from build123d import *

# Parameters (mm, degrees)
SKETCH1_W           = 120
SKETCH1_H           = 120
BOSS_EXTRUDE1_DEPTH = 10
SKETCH2_R           = 45
BOSS_EXTRUDE2_DEPTH = 40
SKETCH3_W           = 10
SKETCH3_H           = 80
BOSS_EXTRUDE3_DEPTH = 50
SKETCH4_R           = 20
BOSS_EXTRUDE4_DEPTH = 25
FILLET1_R           = 2
SKETCH6_R           = 6
BOSS_EXTRUDE5_DEPTH = 2
SKETCH7_R           = 5
BOSS_EXTRUDE6_DEPTH = 30


with BuildPart() as part:
    # Sketch1 → Boss-Extrude1 (new body)
    with BuildSketch(Plane.XY):
        Rectangle(SKETCH1_W, SKETCH1_H)
    extrude(amount=BOSS_EXTRUDE1_DEPTH)

    # Sketch3 → Boss-Extrude3 (add)
    with BuildSketch(Plane(origin=(0, 0, 0), x_dir=(-1, 0, 0), z_dir=(0, 0, -1))):
        with Locations((-25, 0)):
            Rectangle(SKETCH3_W, SKETCH3_H)
        with Locations((25, 0)):
            Rectangle(SKETCH3_W, SKETCH3_H)
    extrude(amount=BOSS_EXTRUDE3_DEPTH)



with BuildPart() as body_2:
    # Sketch2 → Boss-Extrude2 (new body, symmetric)
    with BuildSketch(Plane(origin=(0, 0, 0), x_dir=(1, 0, 0), z_dir=(0, 1, 0))):
        with Locations((0, 50)):
            Circle(SKETCH2_R)
    extrude(amount=BOSS_EXTRUDE2_DEPTH, both=True)


with BuildPart() as part_1:
    add(part.part)

    add(body_2.part)  # Boss-Extrude4 merges body 2
    # Sketch4 → Boss-Extrude4 (add)
    with BuildSketch(Plane(origin=(0, 40, 0), x_dir=(1, 0, 0), z_dir=(0, 1, 0))):
        with Locations((0, 50)):
            Circle(SKETCH4_R)
    extrude(amount=BOSS_EXTRUDE4_DEPTH)

    # Fillet1
    fillet1_edges = [part_1.edges().sort_by_distance(p)[0] for p in [
        (-20, 40, -50),
    ]]
    fillet(fillet1_edges, radius=FILLET1_R)

    # Sketch6 → Boss-Extrude5 (add)
    with BuildSketch(Plane(origin=(0, 65, 0), x_dir=(1, 0, 0), z_dir=(0, 1, 0))):
        with Locations((0, 50)):
            Circle(SKETCH6_R)
    extrude(amount=BOSS_EXTRUDE5_DEPTH)

    # Sketch7 → Boss-Extrude6 (add)
    with BuildSketch(Plane(origin=(0, 67, 0), x_dir=(1, 0, 0), z_dir=(0, 1, 0))):
        with Locations((0, 50)):
            Circle(SKETCH7_R)
    extrude(amount=BOSS_EXTRUDE6_DEPTH)


solid = part_1.part
The listing builds one solid part. Answer for the finished solid, in the listing's coordinates (mm). A direction names the side the tool comes from. Coordinates: 2 decimals unless noted, no trailing zeros. Loops run counter-clockwise (first coordinate to the right, second up) from the corner with the lowest first, then second, coordinate; pieces in that order, holes last. Notation, with made-up numbers: (51.25, 57) -> (64.25, 57) arc R24 ccw to (64.25, 79) -> close; hole circle Ø6 at (76, 58). An arc over 180 degrees is marked (long way). Answer in a Markdown table with one row per item. Add a question column.
1. The part is cut by section D-D, the plane z = -50. Write down the section's boundary in (x, y).
2. Flat-ended cylindrical pins translate along their axes: P1, Ø5, axis at x = -12.5, z = -83.5, coming from the -Y side; P2, Ø3, axis at y = 15.5, z = -81.5, coming from the +X side; P3, Ø10.5, axis at y = 17.5, z = -6.5, coming from the -X side. Find the tip coordinate at first contact, or state that the pin passes through.
3. The part is cut by section C-C, the plane y = 0. Write down the section's boundary in (x, z).
4. Determine the mould class of faces 4 (the cylindrical face through (-1.301, 65.986, -44.143)), 5 (the flat face through (-1, -60, 5)), 6 (the flat face through (20, -1, -5)) for opening direction X: +X half, -X half, draft (parallel to the pull), parting line (faces both ways), or undercut.
5. Consider line 1 (Y direction, x = -34, z = -38.5); line 2 (Z direction, x = -30, y = 43); line 3 (Z direction, x = -31.5, y = -20). Determine where each line is inside the solid, lowest interval first. Write a range as [from, to].
6. The part is cut by section A-A, the plane z = -2.5. Write down the section's boundary in (x, y).
7. For faces 1 (the flat face through (-1, 60, 5)), 2 (the flat face through (4, 65, -55)), 3 (the flat face through (-20, -1, -5)), determine the directions among +Z, -Z, +X, -X, +Y, -Y from which every point of the face is accessible in a straight line to the end or side of a thin tool.
8. The part is cut by section B-B, the plane x = 0. Write down the section's boundary in (y, z).
Answer below:
| question | item | result |
|---|---|---|
| 1 | outline | (-45, -40) -> (45, -40) -> (45, 40) -> (22, 40) arc R2 cw to (20, 42) -> (20, 65) -> (6, 65) -> (6, 67) -> (5, 67) -> (5, 97) -> (-5, 97) -> (-5, 67) -> (-6, 67) -> (-6, 65) -> (-20, 65) -> (-20, 42) arc R2 cw to (-22, 40) -> (-45, 40) -> close |
| 2 | P1 | y = -40 |
| 2 | P2 | x = 33.54 |
| 2 | P3 | x = -30 |
| 3 | outline | (-60, 0) -> (-30, 0) -> (-30, -16.46) arc R45 ccw (long way) to (30, -16.46) -> (30, 0) -> (60, 0) -> (60, 10) -> (-60, 10) -> close; hole (-20, -9.69) arc R45 cw to (20, -9.69) -> (20, 0) -> (-20, 0) -> close |
| 4 | face 4 | parting line |
| 4 | face 5 | draft |
| 4 | face 6 | undercut |
| 5 | line 1 | [-40, 40] |
| 5 | line 2 | [0, 10] |
| 5 | line 3 | [-82.14, -17.86], [0, 10] |
| 6 | outline | (-30, -40) -> (-20, -40) -> (-20, 40) -> (-30, 40) -> close; (20, -40) -> (30, -40) -> (30, 40) -> (20, 40) -> close |
| 7 | face 1 | +Z, +X, -X, +Y |
| 7 | face 2 | +Y |
| 7 | face 3 | +Y, -Y |
| 8 | outline | (-60, 0) -> (60, 0) -> (60, 10) -> (-60, 10) -> close; (-40, -95) -> (40, -95) -> (40, -72) arc R2 cw to (42, -70) -> (65, -70) -> (65, -56) -> (67, -56) -> (67, -55) -> (97, -55) -> (97, -45) -> (67, -45) -> (67, -44) -> (65, -44) -> (65, -30) -> (42, -30) arc R2 cw to (40, -28) -> (40, -5) -> (-40, -5) -> close |
